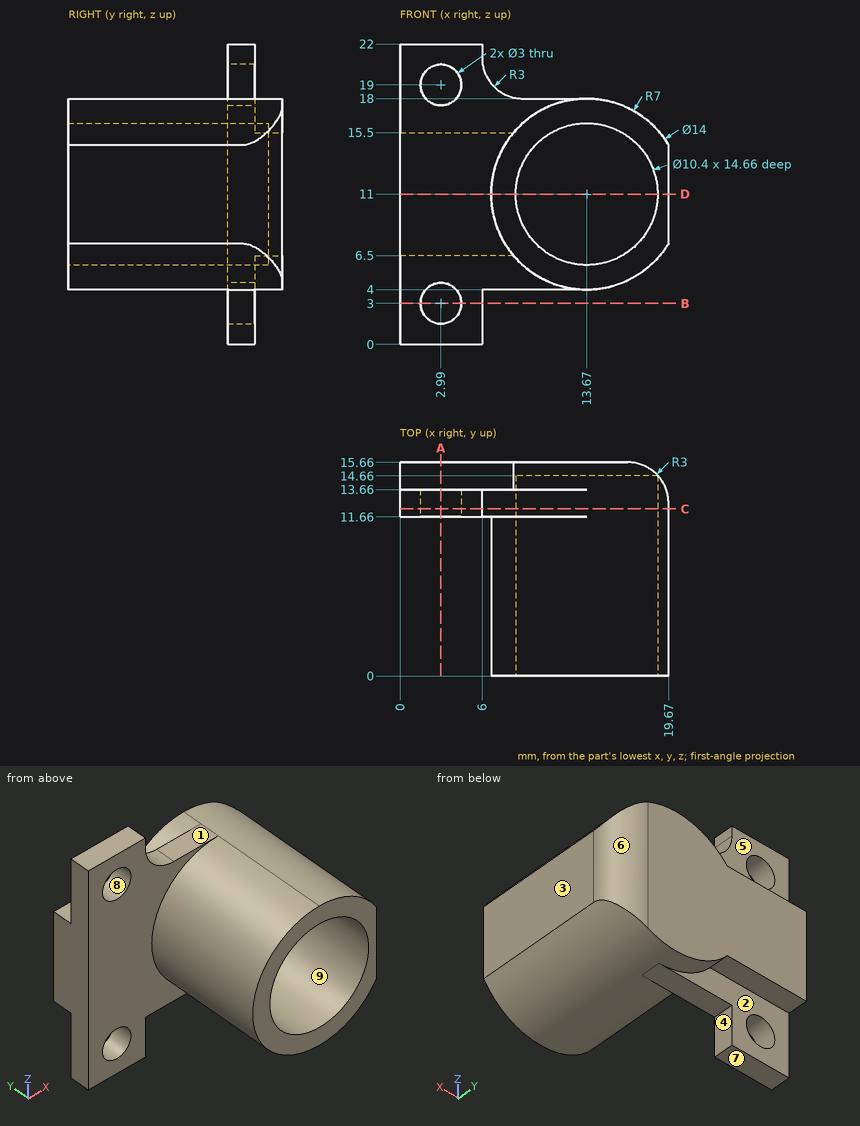
Answer from the drawing. Dimensions are ordinates in mm from the lowest x, y and z of the part. A direction names the side the tool comes from. Coordinates: 2 decimals unless noted, no trailing zeros. Write each loop counter-clockwise with the first axis right and the second up, starting at its lowest first coordinate (ties: lowest second). Pieces come first, ordered by that corner, then holes. Notation, with made-up numbers: M 22,69.25 L 65,69.25 A25 ccw 65,81.25 Z; hole C -29,25.25 d4. An arc over 180 degrees is marked long. Use a Markdown table: item, result.
Q1. The part is cut by section B-B, the plane z = 3. Write down the section's boundary in (x, y), then the cut area to 3 significant figures.
Answer block:
| item | result |
|---|---|
| outline | M 0,11.66 L 1.49,11.66 L 1.49,13.66 L 0,13.66 Z; M 4.49,11.66 L 6,11.66 L 6,13.66 L 4.49,13.66 Z |
| area | 6.00 mm2 |
Q2. The part is cut by section C-C, the plane y = 12.25. Write down the section's boundary in (x, z).
Answer block:
| item | result |
|---|---|
| outline | M 0,0 L 6,0 L 6,4 L 13.67,4 A7 ccw 19.67,7.39 L 19.67,14.61 A7 ccw 13.67,18 L 9,18 A3 cw 6,21 L 6,22 L 0,22 Z; hole C 2.99,3 d3; hole C 2.99,19 d3; hole C 13.67,11 d10.4 |
Q3. Each of these flat-tipped pins is pushed along its axis until it touches: pin 1 Ø1.8 at (x, z) = (2.99, 3) entering from +Y; pin 2 Ø3 at (x, z) = (12, 9.5) entering from -Y; pin 3 Ø2 at (y, z) = (13, 2) entering from +X; pin 4 Ø1.6 at (x, y) = (2.5, 15) entering from +Z. Where does it stop, or does it pass through?
Answer block:
| item | result |
|---|---|
| pin 1 | passes through |
| pin 2 | stops at y = 14.66 |
| pin 3 | stops at x = 6 |
| pin 4 | stops at z = 15.5 |
Q4. The part is cut by section D-D, the plane z = 11. Write down the section's boundary in (x, y), then the cut area to 3 significant figures.
Answer block:
| item | result |
|---|---|
| outline | M 0,11.66 L 6.67,11.66 L 6.67,0 L 8.47,0 L 8.47,14.66 L 18.87,14.66 L 18.87,0 L 19.67,0 L 19.67,12.66 A3 ccw 16.67,15.66 L 0,15.66 Z |
| area | 75.9 mm2 |
Q5. Which of the six approach directions +Z, -Z, +X, -X, +Y, -Y give full straight-line access (tool end or side, diameter ignored) to the marked faces 1, 2, 3, 4 and 5?
Answer block:
| item | result |
|---|---|
| face 1 | +Z, +X, +Y, -Y |
| face 2 | -Z, -X, +Y |
| face 3 | +Z, -Z, +X, +Y, -Y |
| face 4 | -Z, +X, +Y, -Y |
| face 5 | +Z, -X, +Y |
Q6. The part is cut by section A-A, the plane x = 2.99. Write down the section's boundary in (y, z), then the cut area to 3 significant figures.
Answer block:
| item | result |
|---|---|
| outline | M 11.66,0 L 13.66,0 L 13.66,1.5 L 11.66,1.5 Z; M 11.66,4.5 L 13.66,4.5 L 13.66,6.5 L 15.66,6.5 L 15.66,15.5 L 13.66,15.5 L 13.66,17.5 L 11.66,17.5 Z; M 11.66,20.5 L 13.66,20.5 L 13.66,22 L 11.66,22 Z |
| area | 50.0 mm2 |
Q7. Straight lines are drawn through the part: L1, parallel to X at y = 12.2, z = 3; L2, parallel to X at y = 1.5, z = 11; L3, parallel to Y at x = 2.25, z = 9.25. For each, find the intervals that lie inside material, in ascending order. Write a range as [from, to].
Answer block:
| item | result |
|---|---|
| L1 | x = [0, 1.49], [4.49, 6] |
| L2 | x = [6.67, 8.47], [18.87, 19.67] |
| L3 | y = [11.66, 15.66] |
Q8. Determine the mould class of the marked faces 6, 7, 8 and 9 for opening direction Z: released by +Z, released by -Z, zero draft, split by the parting line, or undercut.
Answer block:
| item | result |
|---|---|
| face 6 | zero draft |
| face 7 | released by -Z |
| face 8 | undercut |
| face 9 | undercut |
